from build123d import *

# Parameters (mm, degrees)
SKETCH_1_R               = 25
EXTRUDE_1_DEPTH          = 5
SKETCH_2_R               = 12
EXTRUDE_2_DEPTH          = 13
SKETCH_3_R               = 4
CUT_EXTRUDE_1_DEPTH      = 40.67366885
SKETCH_4_R               = 2.5
CUT_EXTRUDE_2_DEPTH      = 38.669616404
CUT_EXTRUDE_3_DEPTH      = 40.67366885
CUT_EXTRUDE_3_DEPTH_BACK = 40.67366885
SKETCH_5_R               = 2.25
CUT_EXTRUDE_4_DEPTH      = 40.673668895
CUT_EXTRUDE_4_DEPTH_BACK = 40.673668895
SKETCH_6_R               = 2.25


with BuildPart() as part:
    # 草图1 → 凸台-拉伸1 (new body)
    with BuildSketch(Plane(origin=(0, 0, 0), x_dir=(1, 0, 0), z_dir=(0, 1, 0))):
        with Locations(Location((0, 0, 0), (0, 0, 270))):
            Circle(SKETCH_1_R)
    extrude(amount=EXTRUDE_1_DEPTH)

    # 草图2 → 凸台-拉伸2 (add)
    with BuildSketch(Plane(origin=(0, 5, 0), x_dir=(1, 0, 0), z_dir=(0, 1, 0))):
        with Locations(Location((0, 0, 0), (0, 0, 90))):
            Circle(SKETCH_2_R)
    extrude(amount=EXTRUDE_2_DEPTH)

    # 草图3 → 切除-拉伸1 (cut, through all)
    with BuildSketch(Plane(origin=(0, 18, 0), x_dir=(1, 0, 0), z_dir=(0, 1, 0))):
        with Locations(Location((0, 0, 0), (0, 0, 270))):
            Circle(SKETCH_3_R)
    extrude(amount=-CUT_EXTRUDE_1_DEPTH, mode=Mode.SUBTRACT)

    # 草图4 → 切除-拉伸2 (cut, through all)
    with BuildSketch(Plane(origin=(0, 5, 0), x_dir=(1, 0, 0), z_dir=(0, 1, 0))):
        with Locations(Location((0, 18.5, 0), (0, 0, 270))):
            Circle(SKETCH_4_R)
        with Locations(Location((18.5, 0, 0), (0, 0, 270))):
            Circle(SKETCH_4_R)
        with Locations(Location((0, -18.5, 0), (0, 0, 270))):
            Circle(SKETCH_4_R)
        with Locations(Location((-18.5, 0, 0), (0, 0, 270))):
            Circle(SKETCH_4_R)
    extrude(amount=-CUT_EXTRUDE_2_DEPTH, mode=Mode.SUBTRACT)

    # 草图5 → 切除-拉伸3 (cut, two sides: drawn at the far end of the back side and taken through both)
    with BuildSketch(Plane(origin=(0, 0, 0), x_dir=(0, 0, -1), z_dir=(1, 0, 0)).offset(-CUT_EXTRUDE_3_DEPTH_BACK)):
        with Locations((0, 11.5)):
            Circle(SKETCH_5_R)
    extrude(amount=CUT_EXTRUDE_3_DEPTH + CUT_EXTRUDE_3_DEPTH_BACK, mode=Mode.SUBTRACT)

    # 草图6 → 切除-拉伸4 (cut, two sides: drawn at the far end of the back side and taken through both)
    with BuildSketch(Plane.XY.offset(-CUT_EXTRUDE_4_DEPTH_BACK)):
        with Locations((0, 11.5)):
            Circle(SKETCH_6_R)
    extrude(amount=CUT_EXTRUDE_4_DEPTH + CUT_EXTRUDE_4_DEPTH_BACK, mode=Mode.SUBTRACT)


solid = part.part
Verification items for the finished model (mm, model axes). A direction names the side the tool comes from. Give positions to 0.01 mm unless a question says otherwise; leave off trailing zeros. Order: outer loops, then holes, each group sorted by start corner. A loop starts at its lowest first (then second) coordinate and runs counter-clockwise, first axis right, second up. Notation, with made-up numbers: (4.25, 48) -> (47.25, 48) arc R20 cw to (47.25, 65) -> close; hole circle Ø7 at (82, -14). An arc over 180 degrees is marked (long way). Answer as CSV lines item,"result".
Q1. Release check for a two-part mould opening along X. For faces 3 (the cylindrical face through (-0.29, 13.73, -7.71)), 4 (the cylindrical face through (-7.72, 13.73, 0.29)), 5 (the cylindrical face through (10.646, 11.409, -5.537)) record: +X half, -X half, draft (parallel to the pull), parting line (faces both ways), or undercut.
Solutions:
face 3,"undercut"
face 4,"draft"
face 5,"parting line"
Q2. Sectioned sample at D-D on x = 10.5. Record the cut outline in (y, z), plus the area to 3 significant figures.
Solutions:
outline,"(0, -22.69) -> (5, -22.69) -> (5, -5.81) -> (18, -5.81) -> (18, 5.81) -> (5, 5.81) -> (5, 22.69) -> (0, 22.69) -> close; hole circle Ø4.5 at (11.5, 0)"
area,"362 mm²"
Q3. Sectioned sample at B-B on y = 11.5. Record the cut outline in (x, z), plus the area to 3 significant figures.
Solutions:
outline,"(-11.79, -2.25) arc R12 ccw to (-2.25, -11.79) -> (-2.25, -3.31) arc R4 cw to (-3.31, -2.25) -> close; (-11.79, 2.25) -> (-3.31, 2.25) arc R4 cw to (-2.25, 3.31) -> (-2.25, 11.79) arc R12 ccw to start; (2.25, -11.79) arc R12 ccw to (11.79, -2.25) -> (3.31, -2.25) arc R4 cw to (2.25, -3.31) -> close; (2.25, 3.31) arc R4 cw to (3.31, 2.25) -> (11.79, 2.25) arc R12 ccw to (2.25, 11.79) -> close"
area,"255 mm²"
Q4. Access from +Z, -Z, +X, -X, +Y, -Y to the whole of each face (thin tool, end or side, straight path). Record for faces 1 (the flat face through (6, 5, 11)), 2 (the flat face through (-3, 18, 3)).
Solutions:
face 1,"+Y"
face 2,"+Z, -Z, +X, -X, +Y"
Q5. Sectioned sample at C-C on z = -6. Record the cut outline in (x, y), plus the area to 3 significant figures.
Solutions:
outline,"(-24.27, 0) -> (24.27, 0) -> (24.27, 5) -> (10.39, 5) -> (10.39, 18) -> (-10.39, 18) -> (-10.39, 5) -> (-24.27, 5) -> close; hole circle Ø4.5 at (0, 11.5)"
area,"497 mm²"
Q6. Depth check by flat-ended pin: pin 1 (2.5 mm diameter, centred on x = 0, y = 11.5, fed in from -Z); pin 2 (5 mm diameter, centred on y = 11.5, z = 0, fed in from +X); pin 3 (6.5 mm diameter, centred on x = 0, z = -18.5, fed in from +Y); pin 4 (5 mm diameter, centred on x = -7.5, y = 16, fed in from -Z). Enter the tip coordinate at first touch or a pass-through.
Solutions:
pin 1,"passes through"
pin 2,"stops at x = 12"
pin 3,"stops at y = 5"
pin 4,"stops at z = -10.91"
Q7. Sectioned sample at A-A on z = 0. Record the cut outline in (x, y).
Solutions:
outline,"(-25, 0) -> (-21, 0) -> (-21, 5) -> (-25, 5) -> close; (-16, 0) -> (-4, 0) -> (-4, 9.25) -> (-12, 9.25) -> (-12, 5) -> (-16, 5) -> close; (-12, 13.75) -> (-4, 13.75) -> (-4, 18) -> (-12, 18) -> close; (4, 0) -> (16, 0) -> (16, 5) -> (12, 5) -> (12, 9.25) -> (4, 9.25) -> close; (4, 13.75) -> (12, 13.75) -> (12, 18) -> (4, 18) -> close; (21, 0) -> (25, 0) -> (25, 5) -> (21, 5) -> close"
Q8. Scan lines: probe 1 along X at (y, z) = (1.4, 0); probe 2 along Y at (x, z) = (-7, 0); probe 3 along X at (y, z) = (2, -1.5). Record each from-to range of solid material in increasing order.
Solutions:
probe 1,"x = -25 to -21, -16 to -4, 4 to 16, 21 to 25"
probe 2,"y = 0 to 9.25, 13.75 to 18"
probe 3,"x = -24.95 to -20.5, -16.5 to -3.71, 3.71 to 16.5, 20.5 to 24.95"
